The model under review builds one solid part; all positions refer to its coordinate system, in mm. Coordinates: 2 decimals unless noted, no trailing zeros. Write each loop counter-clockwise with the first axis right and the second up, starting at its lowest first coordinate (ties: lowest second). Pieces come first, ordered by that corner, then holes.
```python
from build123d import *

# Parameters (mm, degrees)
SKETCH2_W                = 15
SKETCH2_H                = 5
BOSS_EXTRUDE1_DEPTH      = 5
FILLET2_R                = 1.5
CIRPATTERN4_COUNT        = 3
FILLET2_OF_CIRPATTERN4_R = 1.5


with BuildPart() as part:
    # Sketch2 → Revolve1 (revolve)
    with BuildSketch(Plane(origin=(0, 0, 0), x_dir=(0, 0, -1), z_dir=(1, 0, 0)), mode=Mode.PRIVATE) as revolve1_sk:
        with Locations((-57.5, 2.5)):
            Rectangle(SKETCH2_W, SKETCH2_H)
    revolve(revolve1_sk.sketch.rotate(Axis((0, -0.75, 0), (0, 1, 0)), 180), axis=Axis((0, -0.75, 0), (0, 1, 0)))

    # Sketch4 → Boss-Extrude1 (add)
    with BuildSketch(Plane(origin=(0, 5, 0), x_dir=(1, 0, 0), z_dir=(0, 1, 0))):
        with BuildLine():
            Line((-3.881158746, 64.88402428), (-8.835527397, 71.959595994))
            ThreePointArc((-8.835527397, 71.959595994), (0, 72.5), (8.835527397, 71.959595994))
            Line((8.835527397, 71.959595994), (3.881158746, 64.88402428))
            ThreePointArc((3.881158746, 64.88402428), (0, 65), (-3.881158746, 64.88402428))
        make_face()
    boss_extrude1 = extrude(amount=-BOSS_EXTRUDE1_DEPTH)

    # Fillet2
    fillet2_edges = [part.edges().sort_by_distance(p)[0] for p in [
        (3.881158746, 2.5, -64.88402428),
        (-3.881158746, 2.5, -64.88402428),
        (-8.835527397, 2.5, -71.959595994),
        (8.835527397, 2.5, -71.959595994),
    ]]
    fillet(fillet2_edges, radius=FILLET2_R)

    # CirPattern4: Boss-Extrude1 ×3 about axis
    cirpattern4_axis = Axis((0, 0, 0), (0, 1, 0))
    for i in range(1, CIRPATTERN4_COUNT):
        add(boss_extrude1.rotate(cirpattern4_axis, i * 360 / CIRPATTERN4_COUNT))

    # Fillet2 of CirPattern4
    fillet2_of_cirpattern4_edges = [part.edges().sort_by_distance(p)[0] for p in [
        (-58.131792699, 2.5, 29.08083007),
        (-54.250633954, 2.5, 35.80319421),
        (-57.901074478, 2.5, 43.631589179),
        (-66.736601875, 2.5, 28.328006815),
        (54.250633954, 2.5, 35.80319421),
        (58.131792699, 2.5, 29.08083007),
        (66.736601875, 2.5, 28.328006815),
        (57.901074478, 2.5, 43.631589179),
    ]]
    fillet(fillet2_of_cirpattern4_edges, radius=FILLET2_OF_CIRPATTERN4_R)


solid = part.part
```
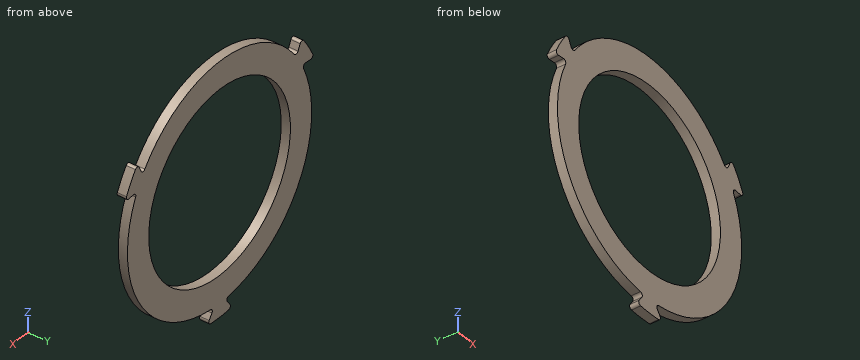
Item 1: For pin 1 (1.5 mm diameter, centred on x = 16, y = 2, fed in from +Z); pin 2 (2 mm diameter, centred on x = 41.5, y = 3, fed in from -Z); pin 3 (1 mm diameter, centred on x = -21, y = 3.5, fed in from +Z), all flat-tipped, find the tip position at first contact; note any pin that passes through.
Solved:
pin 1: stops at z = 63.19
pin 2: stops at z = -50.84
pin 3: stops at z = 61.68
Item 2: Take a section at A-A, the plane z = 0. Write out the cut boundary in (x, y).
Solved:
outline: (-65, 0) - (-50, 0) - (-50, 5) - (-65, 5) - close; (50, 0) - (65, 0) - (65, 5) - (50, 5) - close
Item 3: To check wall thickness, follow line 1 along X through (y, z) = (2.2, 0); line 2 along X through (y, z) = (2.8, -28); line 3 along Z through (x, y) = (8, 0.95). State the ranges of each line that lie inside material, in increasing order.
Solved:
line 1: x = -65 to -50, 50 to 65
line 2: x = -58.66 to -41.42, 41.42 to 58.66
line 3: z = -64.51 to -49.36, 49.36 to 64.51
Item 4: Take a section at C-C, the plane y = 2.8. Write out the cut boundary in (x, z).
Solved:
outline: (-65.69, 30.68) arc R1.5 ccw to (-64.2, 28.55) - (-60.74, 28.85) arc R1.5 cw to (-59.24, 26.74) arc R65 ccw to (-6.46, -64.68) arc R1.5 cw to (-5.38, -67.03) - (-7.37, -69.87) arc R1.5 ccw to (-6.28, -72.23) arc R72.5 ccw to (6.28, -72.23) arc R1.5 ccw to (7.37, -69.87) - (5.38, -67.03) arc R1.5 cw to (6.46, -64.68) arc R65 ccw to (59.24, 26.74) arc R1.5 cw to (60.74, 28.85) - (64.2, 28.55) arc R1.5 ccw to (65.69, 30.68) arc R72.5 ccw to (59.41, 41.55) arc R1.5 ccw to (56.82, 41.32) - (55.36, 38.18) arc R1.5 cw to (52.78, 37.94) arc R65 ccw to (-52.78, 37.94) arc R1.5 cw to (-55.36, 38.18) - (-56.82, 41.32) arc R1.5 ccw to (-59.41, 41.55) arc R72.5 ccw to start; hole circle Ø100 at (0, 0)
Item 5: Take a section at B-B, the plane x = 0. Write out the cut boundary in (y, z), plus the area to 4 significant figures.
Solved:
outline: (0, -72.5) - (5, -72.5) - (5, -50) - (0, -50) - close; (0, 50) - (5, 50) - (5, 65) - (0, 65) - close
area: 187.5 mm2
